```python
from build123d import *

# Parameters (mm, degrees)
SKETCH1_R           = 4.2164
BOSS_EXTRUDE1_DEPTH = 6.35
SKETCH2_R           = 2.5527
CUT_EXTRUDE1_DEPTH  = 6.35
FILLET1_R           = 10


with BuildPart() as part:
    # Sketch1 → Boss-Extrude1 (new body)
    with BuildSketch(Plane.XY):
        Polygon((267.938493178, -135), (219.318011435, -226.869730158), (350, -226.869730158), (350, -135), align=None)
        with Locations((275, -150)):
            Circle(SKETCH1_R, mode=Mode.SUBTRACT)
        with Locations((242.256504613, -211.869730158)):
            Circle(SKETCH1_R, mode=Mode.SUBTRACT)
    extrude(amount=BOSS_EXTRUDE1_DEPTH)

    # Sketch2 → Cut-Extrude1 (cut)
    with BuildSketch(Plane.XY.offset(6.35)):
        with Locations((313.17, -168.234865079)):
            Circle(SKETCH2_R)
        with Locations((338.57, -168.234865079)):
            Circle(SKETCH2_R)
        with Locations((313.17, -193.634865079)):
            Circle(SKETCH2_R)
        with Locations((338.57, -193.634865079)):
            Circle(SKETCH2_R)
    extrude(amount=-CUT_EXTRUDE1_DEPTH, mode=Mode.SUBTRACT)

    # Fillet1
    fillet1_edges = [part.edges().sort_by_distance(p)[0] for p in [
        (350, -135, 3.175),
        (350, -226.869730158, 3.175),
        (219.318011435, -226.869730158, 3.175),
        (267.938493178, -135, 3.175),
    ]]
    fillet(fillet1_edges, radius=FILLET1_R)


solid = part.part
```
Geometry check sheet. Reference: the model listing, model coordinates, mm. Round coordinates to 2 decimals unless told otherwise and drop trailing zeros. Write each loop counter-clockwise with the first axis right and the second up, starting at its lowest first coordinate (ties: lowest second). Pieces come first, ordered by that corner, then holes. Notation, with made-up numbers: (24, 84) -> (74, 84) arc R14 ccw to (74, 88) -> close; hole circle Ø1 at (61, -36.5). An arc over 180 degrees is marked (long way). Put each result on its own line as item: value.
1) Cross-section at B-B, the plane y = -150. Enter the section's corners in (x, z), plus the area to 3 significant figures.
Recorded:
outline: (260, 0) -> (270.78, 0) -> (270.78, 6.35) -> (260, 6.35) -> close; (279.22, 0) -> (350, 0) -> (350, 6.35) -> (279.22, 6.35) -> close
area: 518 mm2
2) Cross-section at D-D, the plane x = 276. Enter the section's corners in (y, z), plus the area to 3 significant figures.
Recorded:
outline: (-226.87, 0) -> (-154.1, 0) -> (-154.1, 6.35) -> (-226.87, 6.35) -> close; (-145.9, 0) -> (-135, 0) -> (-135, 6.35) -> (-145.9, 6.35) -> close
area: 531 mm2
3) Release check for a two-part mould opening along X. For faces 1 (the face through (287, -226.87, 3)), 2 (the face through (246.37, -175.75, 3.13)), 3 (the face through (270.788, -149.815, 3.131)) record: pulls with the +X half, pulls with the -X half, needs draft (parallel to the pull), parting line crosses it, or undercut.
Recorded:
face 1: needs draft
face 2: pulls with the -X half
face 3: undercut
4) Depth check by flat-ended pin: P1, Ø6.5, axis at x = 275, y = -150, coming from the -Z side; P2, Ø1, axis at y = -149.5, z = 4, coming from the -X side; P3, Ø1, axis at y = -178.5, z = 4, coming from the -X side. Enter the tip coordinate at first touch or a pass-through.
Recorded:
P1: passes through
P2: stops at x = 260
P3: stops at x = 244.65
5) Thickness scan on probe 1 along Y at (x, z) = (313.17, 3.25); probe 2 along Y at (x, z) = (273, 5.25); probe 3 along X at (y, z) = (-167.5, 1.5). Record the ranges inside material, lowest first. Write a range as from..to.
Recorded:
probe 1: y = -226.87..-196.19, -191.08..-170.79, -165.68..-135
probe 2: y = -226.87..-153.71, -146.29..-135.05
probe 3: x = 250.74..310.73, 315.61..336.13, 341.01..350
6) Cross-section at C-C, the plane z = 5.25. Enter the section's corners in (x, y), plus the area to 3 significant figures.
Recorded:
outline: (227.09, -212.19) arc R10 ccw to (235.92, -226.87) -> (340, -226.87) arc R10 ccw to (350, -216.87) -> (350, -145) arc R10 ccw to (340, -135) -> (273.96, -135) arc R10 ccw to (265.12, -140.32) -> close; hole circle Ø8.43 at (242.26, -211.87); hole circle Ø8.43 at (275, -150); hole circle Ø5.11 at (313.17, -193.63); hole circle Ø5.11 at (313.17, -168.23); hole circle Ø5.11 at (338.57, -193.63); hole circle Ø5.11 at (338.57, -168.23)
area: 9,470 mm2
7) Cross-section at A-A, the plane x = 313.17. Enter the section's corners in (y, z), plus the area to 3 significant figures.
Recorded:
outline: (-226.87, 0) -> (-196.19, 0) -> (-196.19, 6.35) -> (-226.87, 6.35) -> close; (-191.08, 0) -> (-170.79, 0) -> (-170.79, 6.35) -> (-191.08, 6.35) -> close; (-165.68, 0) -> (-135, 0) -> (-135, 6.35) -> (-165.68, 6.35) -> close
area: 519 mm2
